Here's how the part is built. I have some questions about the finished solid (model axes, mm). Round coordinates to 2 decimals unless told otherwise and drop trailing zeros. Write each loop counter-clockwise with the first axis right and the second up, starting at its lowest first coordinate (ties: lowest second). Pieces come first, ordered by that corner, then holes. Notation, with made-up numbers: (86.5, 2.25) - (98.5, 2.25) arc R27 ccw to (98.5, 35.25) - close; hole circle Ø1 at (-37, 67). An arc over 180 degrees is marked (long way). Write item = value, one per line. Start each with the question number.
Item 1: If we section it at A-A (z = 59.5): Please give me the cut outline in (x, y).
Item 2: If we section it at B-B (x = -4.5): Give the number of separate pieces and of enclosed holes in the cut face, and give its area (3 significant figures).
Item 3: For P1, Ø3, axis at x = -3.5, z = 126, coming from the +Y side; P2, Ø3, axis at x = -4.5, z = 106.94, coming from the +Y side (1 decimal), each with a flat end and sliding along its axis, tell me the tip position at first contact or that it passes through.
Item 4: If I drill on line 1 along Y through (x, z) = (-8.25, 51.5); line 2 along X through (y, z) = (3.75, 46.5); line 3 along X through (y, z) = (2.75, 247), over which ranges is the centre line in solid material (lowest first)? Write a range as [from, to].
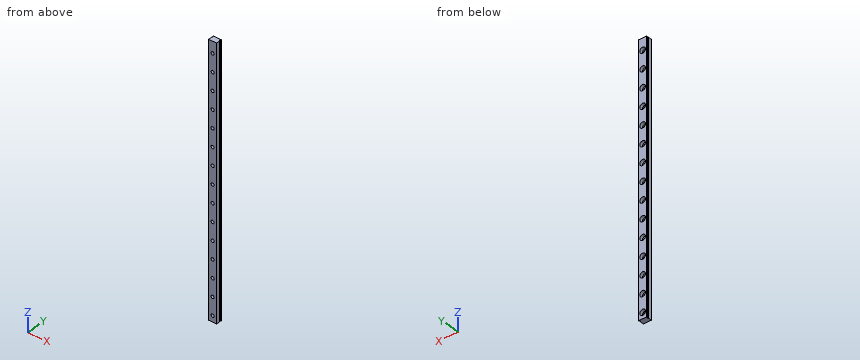
```python
from build123d import *

# Parameters (mm, degrees)
EXTRUDE_1_DEPTH     = 300
SKETCH_2_R          = 1.75
CUT_EXTRUDE_3_DEPTH = 440
SKETCH_3_R          = 3.25
CUT_EXTRUDE_4_DEPTH = 3.5


with BuildPart() as part:
    # 草图1 → 凸台-拉伸1 (new body)
    with BuildSketch(Plane.XY):
        Polygon((0, 0), (-9, 0), (-9, 4.208125846), (-8.343397225, 4.785997189), (-8.055092033, 4.785997189), (-8.055092033, 5.184529149), (-8.343397225, 5.184529149), (-9, 5.762400492), (-9, 6.5), (0, 6.5), (0, 5.762400492), (-0.656602775, 5.184529149), (-0.944907967, 5.184529149), (-0.944907967, 4.785997189), (-0.656602775, 4.785997189), (0, 4.208125846), align=None)
    extrude(amount=EXTRUDE_1_DEPTH)

    # 草图2 → 切除-拉伸3 (cut)
    with BuildSketch(Plane(origin=(0, 6.5, 0), x_dir=(1, 0, 0), z_dir=(0, 1, 0))):
        with Locations(Location((-4.5, -6.942433545, 0), (0, 0, 180))):
            Circle(SKETCH_2_R)
        with Locations(Location((-4.5, -26.942433545, 0), (0, 0, 180))):
            Circle(SKETCH_2_R)
        with Locations(Location((-4.5, -46.942433545, 0), (0, 0, 180))):
            Circle(SKETCH_2_R)
        with Locations(Location((-4.5, -66.942433545, 0), (0, 0, 180))):
            Circle(SKETCH_2_R)
        with Locations(Location((-4.5, -86.942433545, 0), (0, 0, 180))):
            Circle(SKETCH_2_R)
        with Locations(Location((-4.5, -106.942433545, 0), (0, 0, 180))):
            Circle(SKETCH_2_R)
        with Locations(Location((-4.5, -126.942433545, 0), (0, 0, 180))):
            Circle(SKETCH_2_R)
        with Locations(Location((-4.5, -146.942433545, 0), (0, 0, 180))):
            Circle(SKETCH_2_R)
        with Locations(Location((-4.5, -166.942433545, 0), (0, 0, 180))):
            Circle(SKETCH_2_R)
        with Locations(Location((-4.5, -186.942433545, 0), (0, 0, 180))):
            Circle(SKETCH_2_R)
        with Locations(Location((-4.5, -206.942433545, 0), (0, 0, 180))):
            Circle(SKETCH_2_R)
        with Locations(Location((-4.5, -226.942433545, 0), (0, 0, 180))):
            Circle(SKETCH_2_R)
        with Locations(Location((-4.5, -246.942433545, 0), (0, 0, 180))):
            Circle(SKETCH_2_R)
        with Locations(Location((-4.5, -266.942433545, 0), (0, 0, 180))):
            Circle(SKETCH_2_R)
        with Locations(Location((-4.5, -286.942433545, 0), (0, 0, 180))):
            Circle(SKETCH_2_R)
        with Locations((-4.5, -306.942433545)):
            Circle(SKETCH_2_R)
        with Locations((-4.5, -326.942433545)):
            Circle(SKETCH_2_R)
        with Locations((-4.5, -346.942433545)):
            Circle(SKETCH_2_R)
        with Locations((-4.5, -366.942433545)):
            Circle(SKETCH_2_R)
        with Locations((-4.5, -386.942433545)):
            Circle(SKETCH_2_R)
        with Locations((-4.5, -406.942433545)):
            Circle(SKETCH_2_R)
        with Locations((-4.5, -426.942433545)):
            Circle(SKETCH_2_R)
    extrude(amount=-CUT_EXTRUDE_3_DEPTH, mode=Mode.SUBTRACT)

    # 草图3 → 切除-拉伸4 (cut)
    with BuildSketch(Plane(origin=(0, 6.5, 0), x_dir=(1, 0, 0), z_dir=(0, 1, 0))):
        with Locations(Location((-4.5, -6.942433545, 0), (0, 0, 180))):
            Circle(SKETCH_3_R)
        with Locations(Location((-4.5, -26.942433545, 0), (0, 0, 180))):
            Circle(SKETCH_3_R)
        with Locations(Location((-4.5, -46.942433545, 0), (0, 0, 180))):
            Circle(SKETCH_3_R)
        with Locations(Location((-4.5, -66.942433545, 0), (0, 0, 180))):
            Circle(SKETCH_3_R)
        with Locations(Location((-4.5, -86.942433545, 0), (0, 0, 180))):
            Circle(SKETCH_3_R)
        with Locations(Location((-4.5, -106.942433545, 0), (0, 0, 180))):
            Circle(SKETCH_3_R)
        with Locations(Location((-4.5, -126.942433545, 0), (0, 0, 180))):
            Circle(SKETCH_3_R)
        with Locations(Location((-4.5, -146.942433545, 0), (0, 0, 180))):
            Circle(SKETCH_3_R)
        with Locations(Location((-4.5, -166.942433545, 0), (0, 0, 180))):
            Circle(SKETCH_3_R)
        with Locations(Location((-4.5, -186.942433545, 0), (0, 0, 180))):
            Circle(SKETCH_3_R)
        with Locations(Location((-4.5, -206.942433545, 0), (0, 0, 180))):
            Circle(SKETCH_3_R)
        with Locations(Location((-4.5, -226.942433545, 0), (0, 0, 180))):
            Circle(SKETCH_3_R)
        with Locations(Location((-4.5, -246.942433545, 0), (0, 0, 180))):
            Circle(SKETCH_3_R)
        with Locations(Location((-4.5, -266.942433545, 0), (0, 0, 180))):
            Circle(SKETCH_3_R)
        with Locations(Location((-4.5, -286.942433545, 0), (0, 0, 180))):
            Circle(SKETCH_3_R)
        with Locations((-4.5, -306.942433545)):
            Circle(SKETCH_3_R)
        with Locations((-4.5, -326.942433545)):
            Circle(SKETCH_3_R)
        with Locations((-4.5, -346.942433545)):
            Circle(SKETCH_3_R)
        with Locations((-4.5, -366.942433545)):
            Circle(SKETCH_3_R)
        with Locations((-4.5, -386.942433545)):
            Circle(SKETCH_3_R)
        with Locations((-4.5, -406.942433545)):
            Circle(SKETCH_3_R)
        with Locations((-4.5, -426.942433545)):
            Circle(SKETCH_3_R)
        with Locations((-4.5, -446.942433545)):
            Circle(SKETCH_3_R)
        with Locations((-4.5, -466.942433545)):
            Circle(SKETCH_3_R)
        with Locations((-4.5, -486.942433545)):
            Circle(SKETCH_3_R)
        with Locations((-4.5, -506.942433545)):
            Circle(SKETCH_3_R)
        with Locations((-4.5, -526.942433545)):
            Circle(SKETCH_3_R)
        with Locations((-4.5, -546.942433545)):
            Circle(SKETCH_3_R)
        with Locations((-4.5, -566.942433545)):
            Circle(SKETCH_3_R)
        with Locations((-4.5, -586.942433545)):
            Circle(SKETCH_3_R)
        with Locations((-4.5, -606.942433545)):
            Circle(SKETCH_3_R)
    extrude(amount=-CUT_EXTRUDE_4_DEPTH, mode=Mode.SUBTRACT)


solid = part.part
```
Reply:
q1.outline = (-9, 0) - (0, 0) - (0, 4.21) - (-0.66, 4.79) - (-0.94, 4.79) - (-0.94, 5.18) - (-0.66, 5.18) - (0, 5.76) - (0, 6.5) - (-9, 6.5) - (-9, 5.76) - (-8.34, 5.18) - (-8.06, 5.18) - (-8.06, 4.79) - (-8.34, 4.79) - (-9, 4.21) - close
q2.separate_pieces = 16
q2.enclosed_holes = 0
q2.area = 1,450 mm2
q3.P1 = 3
q3.P2 = through
q4.line_1 = [0, 4.79], [5.18, 6.5]
q4.line_2 = [-9, -7.72], [-1.28, 0]
q4.line_3 = [-9, -6.25], [-2.75, 0]
